Verification items for the finished model (mm, model axes). Round coordinates to 2 decimals unless told otherwise and drop trailing zeros. Loops run counter-clockwise (first coordinate to the right, second up) from the corner with the lowest first, then second, coordinate; pieces in that order, holes last. Notation, with made-up numbers: M 55,78.5 L 63,78.5 A18 cw 63,110.5 Z; hole C 73,43.25 d2. An arc over 180 degrees is marked long. One line per item, written item: value.
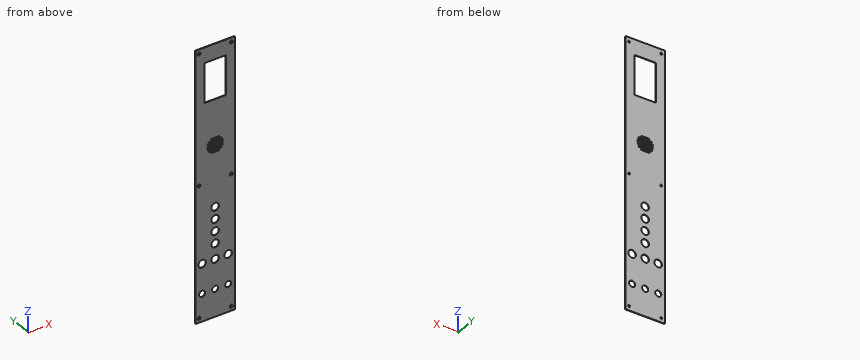
from build123d import *

# Parameters (mm, degrees)
F0_W     = 180
F0_H     = 1230
F0_R     = 3
F0_R_2   = 14
F0_R_3   = 17.5
F0_W_2   = 98
F0_H_2   = 180
F1_DEPTH = 2.5


# Not quite as in the source:
# - a fillet or chamfer that OpenCascade refuses, or shapes differently, is made with other operations: its cross-section is extruded or revolved along the edge and cut away or added
# - the program builds the solid bodies; features that only make, move or delete a surface that nothing else refers to are left out


with BuildPart() as f1:
    # F0 (on Front) → F1 (new body)
    with BuildSketch(Plane.XZ):
        with Locations((-49, -0.441852957)):
            Rectangle(F0_W, F0_H)
        with Locations((-123, -595.441852957)):
            Circle(F0_R, mode=Mode.SUBTRACT)
        with Locations((-109, -490.441852957)):
            Circle(F0_R_2, mode=Mode.SUBTRACT)
        with Locations((-109, -355.441852957)):
            Circle(F0_R_3, mode=Mode.SUBTRACT)
        with Locations((-49, -490.441852957)):
            Circle(F0_R_2, mode=Mode.SUBTRACT)
        with Locations((-49, -355.441852957)):
            Circle(F0_R_3, mode=Mode.SUBTRACT)
        with Locations((11, -490.441852957)):
            Circle(F0_R_2, mode=Mode.SUBTRACT)
        with Locations((25, -595.441852957)):
            Circle(F0_R, mode=Mode.SUBTRACT)
        with Locations((11, -355.441852957)):
            Circle(F0_R_3, mode=Mode.SUBTRACT)
        with Locations((-49, -285.441852957)):
            Circle(F0_R_3, mode=Mode.SUBTRACT)
        with Locations((-49, -230.441852957)):
            Circle(F0_R_3, mode=Mode.SUBTRACT)
        with Locations((-49, -175.441852957)):
            Circle(F0_R_3, mode=Mode.SUBTRACT)
        with Locations((-49, -120.441852957)):
            Circle(F0_R_3, mode=Mode.SUBTRACT)
        with Locations((-123, 0.558147043)):
            Circle(F0_R, mode=Mode.SUBTRACT)
        with BuildLine():
            Line((-30.9722436227, 127.558147043), (-67.0277563773, 127.558147043))
            ThreePointArc((-67.0277563773, 127.558147043), (-69.0277563773, 129.558147043), (-67.0277563773, 131.558147043))
            Line((-67.0277563773, 131.558147043), (-30.9722436227, 131.558147043))
            ThreePointArc((-30.9722436227, 131.558147043), (-28.9722436227, 129.558147043), (-30.9722436227, 127.558147043))
        make_face(mode=Mode.SUBTRACT)
        with BuildLine():
            Line((-20.2771867673, 137.558147043), (-77.7228132327, 137.558147043))
            ThreePointArc((-77.7228132327, 137.558147043), (-79.7228132327, 139.558147043), (-77.7228132327, 141.558147043))
            Line((-77.7228132327, 141.558147043), (-20.2771867673, 141.558147043))
            ThreePointArc((-20.2771867673, 141.558147043), (-18.2771867673, 139.558147043), (-20.2771867673, 137.558147043))
        make_face(mode=Mode.SUBTRACT)
        with BuildLine():
            Line((-15.4589803375, 147.558147043), (-82.5410196625, 147.558147043))
            ThreePointArc((-82.5410196625, 147.558147043), (-84.5410196625, 149.558147043), (-82.5410196625, 151.558147043))
            Line((-82.5410196625, 151.558147043), (-15.4589803375, 151.558147043))
            ThreePointArc((-15.4589803375, 151.558147043), (-13.4589803375, 149.558147043), (-15.4589803375, 147.558147043))
        make_face(mode=Mode.SUBTRACT)
        with BuildLine():
            Line((-15.4589803375, 167.558147043), (-82.5410196625, 167.558147043))
            ThreePointArc((-82.5410196625, 167.558147043), (-84.5410196625, 169.558147043), (-82.5410196625, 171.558147043))
            Line((-82.5410196625, 171.558147043), (-15.4589803375, 171.558147043))
            ThreePointArc((-15.4589803375, 171.558147043), (-13.4589803375, 169.558147043), (-15.4589803375, 167.558147043))
        make_face(mode=Mode.SUBTRACT)
        with BuildLine():
            Line((-20.2771867673, 177.558147043), (-77.7228132327, 177.558147043))
            ThreePointArc((-77.7228132327, 177.558147043), (-79.7228132327, 179.558147043), (-77.7228132327, 181.558147043))
            Line((-77.7228132327, 181.558147043), (-20.2771867673, 181.558147043))
            ThreePointArc((-20.2771867673, 181.558147043), (-18.2771867673, 179.558147043), (-20.2771867673, 177.558147043))
        make_face(mode=Mode.SUBTRACT)
        with BuildLine():
            Line((-30.9722436227, 187.558147043), (-67.0277563773, 187.558147043))
            ThreePointArc((-67.0277563773, 187.558147043), (-69.0277563773, 189.558147043), (-67.0277563773, 191.558147043))
            Line((-67.0277563773, 191.558147043), (-30.9722436227, 191.558147043))
            ThreePointArc((-30.9722436227, 191.558147043), (-28.9722436227, 189.558147043), (-30.9722436227, 187.558147043))
        make_face(mode=Mode.SUBTRACT)
        with Locations((-123, 594.558147043)):
            Circle(F0_R, mode=Mode.SUBTRACT)
        with BuildLine():
            Line((-14, 157.558147043), (-84, 157.558147043))
            ThreePointArc((-84, 157.558147043), (-86, 159.558147043), (-84, 161.558147043))
            Line((-84, 161.558147043), (-14, 161.558147043))
            ThreePointArc((-14, 161.558147043), (-12, 159.558147043), (-14, 157.558147043))
        make_face(mode=Mode.SUBTRACT)
        with Locations((25, 0.558147043)):
            Circle(F0_R, mode=Mode.SUBTRACT)
        with Locations((-49, 454.558147043)):
            Rectangle(F0_W_2, F0_H_2, mode=Mode.SUBTRACT)
        with Locations((25, 594.558147043)):
            Circle(F0_R, mode=Mode.SUBTRACT)
    extrude(amount=F1_DEPTH)

    # F2: chamfer of 4 on 6 edges, made by hand

    # F2_s1 → F2_t2 (revolve, cut)
    with BuildSketch(Plane.XY.offset(-595.441852957)):
        Polygon((28, 1.5), (32, -2.5), (28, -2.5), align=None)
    revolve(axis=Axis((25, -2.5, -595.441852957), (0, -1, 0)), mode=Mode.SUBTRACT)

    # F2_s3 → F2_t4 (revolve, cut)
    with BuildSketch(Plane.XY.offset(-595.441852957)):
        Polygon((-120, 1.5), (-116, -2.5), (-120, -2.5), align=None)
    revolve(axis=Axis((-123, -2.5, -595.441852957), (0, -1, 0)), mode=Mode.SUBTRACT)

    # F2_s5 → F2_t6 (revolve, cut)
    with BuildSketch(Plane.XY.offset(0.558147043)):
        Polygon((-120, 1.5), (-116, -2.5), (-120, -2.5), align=None)
    revolve(axis=Axis((-123, -2.5, 0.558147043), (0, -1, 0)), mode=Mode.SUBTRACT)

    # F2_s7 → F2_t8 (revolve, cut)
    with BuildSketch(Plane.XY.offset(0.558147043)):
        Polygon((28, 1.5), (32, -2.5), (28, -2.5), align=None)
    revolve(axis=Axis((25, -2.5, 0.558147043), (0, -1, 0)), mode=Mode.SUBTRACT)

    # F2_s9 → F2_t10 (revolve, cut)
    with BuildSketch(Plane.XY.offset(594.558147043)):
        Polygon((28, 1.5), (32, -2.5), (28, -2.5), align=None)
    revolve(axis=Axis((25, -2.5, 594.558147043), (0, -1, 0)), mode=Mode.SUBTRACT)

    # F2_s11 → F2_t12 (revolve, cut)
    with BuildSketch(Plane.XY.offset(594.558147043)):
        Polygon((-120, 1.5), (-116, -2.5), (-120, -2.5), align=None)
    revolve(axis=Axis((-123, -2.5, 594.558147043), (0, -1, 0)), mode=Mode.SUBTRACT)


solid = f1.part
(1) Sectioned sample at A-A on z = 383. Enter the section's corners in (x, y).
Completed:
outline: M -139,-2.5 L -98,-2.5 L -98,0 L -139,0 Z; M 0,-2.5 L 41,-2.5 L 41,0 L 0,0 Z
(2) Thickness scan on L1, parallel to Z at x = 11, y = -0.6; L2, parallel to Z at x = -16, y = -1.8; L3, parallel to Z at x = -86.5, y = -1. Record the ranges inside material, lowest first. Write a range as from..to.
Completed:
L1: z = -615.44..-504.44, -476.44..-372.94, -337.94..614.56
L2: z = -615.44..147.56, 151.56..157.56, 161.56..167.56, 171.56..364.56, 544.56..614.56
L3: z = -615.44..364.56, 544.56..614.56
(3) Sectioned sample at B-B on x = -49. Count the separate pieces of the cut face and the enclosed holes in it, and give its area (3 significant figures).
Completed:
separate pieces: 15
enclosed holes: 0
area: 2,050 mm^2
